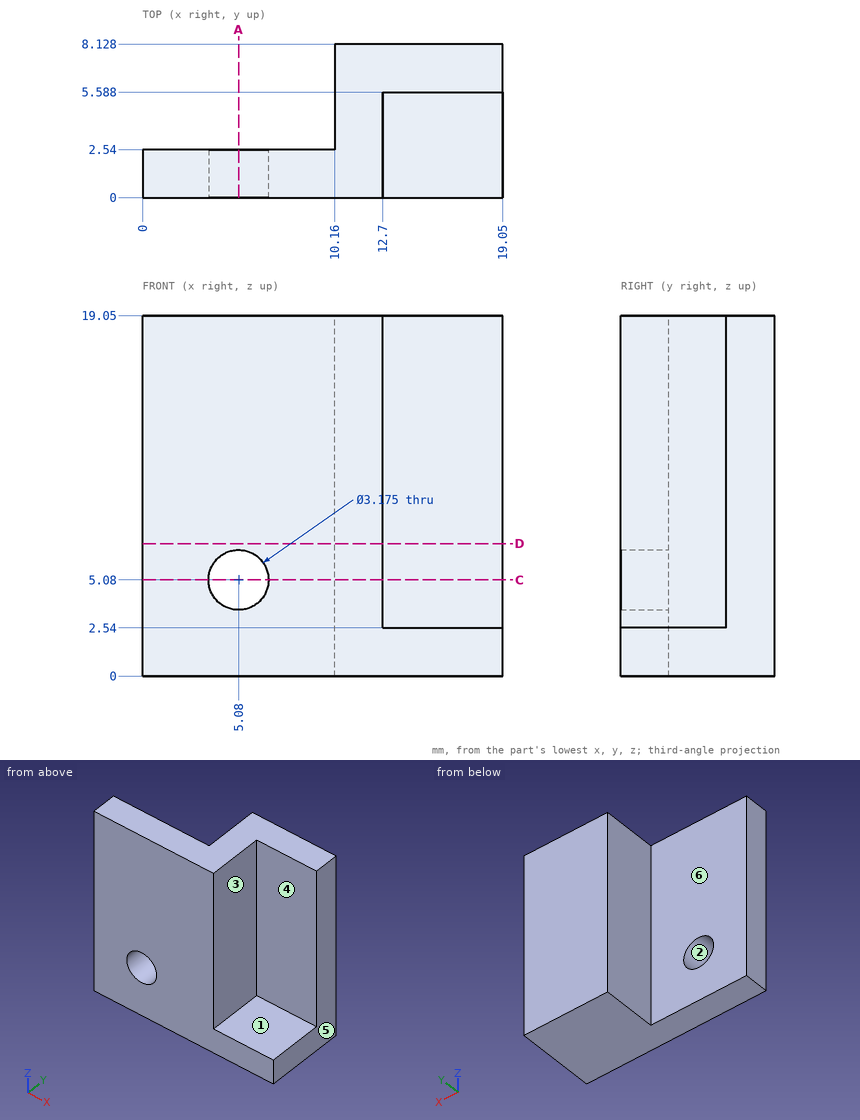
Check sheet for the drawn part. Datum: minimum x, y, z corner. Units: mm. A direction names the side the tool comes from. Round coordinates to 2 decimals unless told otherwise and drop trailing zeros. Order: outer loops, then holes, each group sorted by start corner. A loop starts at its lowest first (then second) coordinate and runs counter-clockwise, first axis right, second up. Notation, with made-up numbers: (5, 38) -> (10, 38) arc R3 ccw to (10, 42) -> close; hole circle Ø8 at (-23.75, 61). An arc over 180 degrees is marked (long way). Put each result on its own line as item: value.
1) Section check D-D (z = 7). Record the cut outline in (x, y), then the cut area to 3 significant figures.
Final values:
outline: (0, 0) -> (12.7, 0) -> (12.7, 5.59) -> (19.05, 5.59) -> (19.05, 8.13) -> (10.16, 8.13) -> (10.16, 2.54) -> (0, 2.54) -> close
area: 62.6 mm^2
2) Section check A-A (x = 5.08). Record the cut outline in (y, z).
Final values:
outline: (0, 0) -> (2.54, 0) -> (2.54, 3.49) -> (0, 3.49) -> close; (0, 6.67) -> (2.54, 6.67) -> (2.54, 19.05) -> (0, 19.05) -> close
3) Depth check by flat-ended pin: pin 1 (5 mm diameter, centred on x = 3, z = 7, fed in from +Y); pin 2 (1.7 mm diameter, centred on x = 16.5, y = 3, fed in from +Z); pin 3 (3 mm diameter, centred on x = 5.08, z = 5.08, fed in from -Y). Enter the tip coordinate at first touch or a pass-through.
Final values:
pin 1: stops at y = 2.54
pin 2: stops at z = 2.54
pin 3: passes through
4) Set-up check for the marked faces 4, 5 and 6: record each of +Z, -Z, +X, -X, +Y, -Y from which the full face is reachable in a straight line by a thin tool's end or side.
Final values:
face 4: +Z, +X, -Y
face 5: +Z, -Z, +X, +Y, -Y
face 6: +Z, -Z, -X, +Y
5) Material ranges on line 1 (Z direction, x = 5.08, y = 1.15); line 2 (X direction, y = 5.5, z = 14.25); line 3 (Y direction, x = 3.25, z = 2.5), recorded low to high.
Final values:
line 1: z = 0 to 3.49, 6.67 to 19.05
line 2: x = 10.16 to 12.7
line 3: y = 0 to 2.54
6) Section check C-C (z = 5.08). Record the cut outline in (x, y).
Final values:
outline: (0, 0) -> (3.49, 0) -> (3.49, 2.54) -> (0, 2.54) -> close; (6.67, 0) -> (12.7, 0) -> (12.7, 5.59) -> (19.05, 5.59) -> (19.05, 8.13) -> (10.16, 8.13) -> (10.16, 2.54) -> (6.67, 2.54) -> close
7) Mould release check, pull along Z, two halves, no side actions. Record for the marked faces 1, 2 and 3: +Z half, -Z half, draft (parallel to the pull), parting line (faces both ways), or undercut.
Final values:
face 1: +Z half
face 2: undercut
face 3: draft
